```python
from build123d import *

# Parameters (mm, degrees)
SKETCH1_W           = 22
SKETCH1_H           = 13
BOSS_EXTRUDE1_DEPTH = 6
BOSS_EXTRUDE2_DEPTH = 2
BOSS_EXTRUDE3_DEPTH = 8
SKETCH4_R           = 1.525
SKETCH4_R_2         = 1.524
CUT_EXTRUDE1_DEPTH  = 36.566838488
SKETCH5_W           = 9
SKETCH5_H           = 4.088652256
CUT_EXTRUDE2_DEPTH  = 38.735924528
FILLET1_R           = 2
SKETCH6_W           = 12
SKETCH6_H           = 13.009000019
SKETCH6_W_2         = 15.838286437
CUT_EXTRUDE3_DEPTH  = 4
SKETCH7_W           = 2.5
SKETCH7_H           = 8
BOSS_EXTRUDE5_DEPTH = 3
FILLET3_R           = 2.5
FILLET4_R           = 2.5


with BuildPart() as part:
    # Sketch1 → Boss-Extrude1 (new body)
    with BuildSketch(Plane(origin=(0, 0, 0), x_dir=(1, 0, 0), z_dir=(0, 1, 0))):
        with BuildLine():
            Line((-1, -3), (23, -3))
            Line((23, -3), (25, -3))
            Line((25, -3), (25, -1))
            Line((25, -1), (25, 14))
            Line((25, 14), (25, 16))
            Line((25, 16), (23, 16))
            Line((23, 16), (-1, 16))
            ThreePointArc((-1, 16), (-2.414213562, 15.414213562), (-3, 14))
            Line((-3, 14), (-3, -1))
            ThreePointArc((-3, -1), (-2.414213562, -2.414213562), (-1, -3))
        make_face()
        with Locations((11, 6.5)):
            Rectangle(SKETCH1_W, SKETCH1_H, mode=Mode.SUBTRACT)
    extrude(amount=BOSS_EXTRUDE1_DEPTH)

    # Sketch2 → Boss-Extrude2 (add)
    with BuildSketch(Plane(origin=(0, 6, 0), x_dir=(1, 0, 0), z_dir=(0, 1, 0))):
        with BuildLine():
            Line((25, 14), (25, -1))
            Line((25, -1), (25, -3))
            Line((25, -3), (23, -3))
            Line((23, -3), (-1, -3))
            ThreePointArc((-1, -3), (-2.414213562, -2.414213562), (-3, -1))
            Line((-3, -1), (-3, 14))
            ThreePointArc((-3, 14), (-2.414213562, 15.414213562), (-1, 16))
            Line((-1, 16), (23, 16))
            Line((23, 16), (25, 16))
            Line((25, 16), (25, 14))
        make_face()
    extrude(amount=BOSS_EXTRUDE2_DEPTH)

    # Sketch3 → Boss-Extrude3 (add)
    with BuildSketch(Plane.XZ):
        with BuildLine():
            Line((5, 3), (17, 3))
            Line((17, 3), (17, 5.5))
            ThreePointArc((17, 5.5), (15.389087297, 9.389087297), (11.5, 11))
            Line((11.5, 11), (10.5, 11))
            ThreePointArc((10.5, 11), (6.610912703, 9.389087297), (5, 5.5))
            Line((5, 5.5), (5, 3))
        make_face()
        with BuildLine():
            Line((17, -16), (5, -16))
            Line((5, -16), (5, -18.5))
            ThreePointArc((5, -18.5), (6.610912703, -22.389087297), (10.5, -24))
            Line((10.5, -24), (11.5, -24))
            ThreePointArc((11.5, -24), (15.389087297, -22.389087297), (17, -18.5))
            Line((17, -18.5), (17, -16))
        make_face()
    extrude(amount=-BOSS_EXTRUDE3_DEPTH)

    # Sketch4 → Cut-Extrude1 (cut, through all)
    with BuildSketch(Plane(origin=(0, 0, 0), x_dir=(-1, 0, 0), z_dir=(0, -1, 0))):
        with Locations(Location((-11, 20, 0), (0, 0, 90))):
            Circle(SKETCH4_R)
        with Locations(Location((-11, -7, 0), (0, 0, 90))):
            Circle(SKETCH4_R_2)
    extrude(amount=-CUT_EXTRUDE1_DEPTH, mode=Mode.SUBTRACT)

    # Sketch5 → Cut-Extrude2 (cut, through all)
    with BuildSketch(Plane(origin=(25, 0, 0), x_dir=(0, 0, -1), z_dir=(1, 0, 0))):
        with Locations((6.5, 2.044326128)):
            Rectangle(SKETCH5_W, SKETCH5_H)
    extrude(amount=-CUT_EXTRUDE2_DEPTH, mode=Mode.SUBTRACT)

    # Fillet1
    fillet1_edges = [part.edges().sort_by_distance(p)[0] for p in [
        (-1.5, 4.088652256, -11),
        (-1.5, 4.088652256, -2),
        (23.5, 4.088652256, -11),
        (23.5, 4.088652256, -2),
    ]]
    fillet(fillet1_edges, radius=FILLET1_R)

    # Sketch6 → Cut-Extrude3 (cut)
    with BuildSketch(Plane(origin=(0, 8, 0), x_dir=(1, 0, 0), z_dir=(0, 1, 0))):
        with Locations((11, 22.504500009)):
            Rectangle(SKETCH6_W, SKETCH6_H)
        with Locations((11.149066226, -9.50450001)):
            Rectangle(SKETCH6_W_2, SKETCH6_H)
    extrude(amount=-CUT_EXTRUDE3_DEPTH, mode=Mode.SUBTRACT)

    # Sketch7 → Boss-Extrude5 (add)
    with BuildSketch(Plane(origin=(25, 0, 0), x_dir=(0, 0, -1), z_dir=(1, 0, 0))):
        with Locations((17.25, 4)):
            Rectangle(SKETCH7_W, SKETCH7_H)
        with Locations((-4.25, 4)):
            Rectangle(SKETCH7_W, SKETCH7_H)
    extrude(amount=-BOSS_EXTRUDE5_DEPTH)

    # Fillet3
    fillet3_edges = [part.edges().sort_by_distance(p)[0] for p in [
        (22, 4, -16),
    ]]
    fillet(fillet3_edges, radius=FILLET3_R - 0.0001)  # a hair under: the kernel refuses the full size

    # Fillet4
    fillet4_edges = [part.edges().sort_by_distance(p)[0] for p in [
        (22, 4, 3),
    ]]
    fillet(fillet4_edges, radius=FILLET4_R - 0.0001)  # a hair under: the kernel refuses the full size


solid = part.part
```
Could you check a few things on this model? Use its own coordinates, in mm. A direction names the side the tool comes from. Give positions to 0.01 mm unless a question says otherwise; leave off trailing zeros. Order: outer loops, then holes, each group sorted by start corner. A loop starts at its lowest first (then second) coordinate and runs counter-clockwise, first axis right, second up.
Q1. I'm going to push flat-ended pins straight in: P1, Ø0.6, axis at x = 23.5, y = 0.5, coming from the -Z side; P2, Ø2.5, axis at x = 11, z = 7, coming from the +Y side; P3, Ø1.5, axis at x = 1, y = 3, coming from the +Z side; P4, Ø1, axis at y = 6, z = 4, coming from the -X side. Where does each tip first touch, or does it pass through?
Q2. Suppose I cut it at C-C, the plane z = -20. Write out the boundary of the cut face in (x, y) (1 decimal).
Q3. Suppose I cut it at A-A, the plane x = 11. Write out the boundary of the cut face in (y, z) (3 decimals).
Q4. If I drill on line 1 along Z through (x, y) = (11.5, 4.25); line 2 along Z through (x, y) = (10, 0.75); line 3 along Z through (x, y) = (-0.5, 5.75), over which ranges is the centre line in solid material (lowest first)?
Q5. Suppose I cut it at D-D, the plane y = 1.25. Count the separate pieces of the cut face and the enclosed holes in it, and give its area (3 significant figures).
Q6. For faces 5 (the flat face through (9.58, 4, 6.06)), 6 (the flat face through (24, 4.089, -6)), 7 (the flat face through (17, 2, -17)), 8 (the flat face through (24, 4, -18.5)), which set-ups out of +Z, -Z, +X, -X, +Y, -Y let a thin tool reach every point of the face, with its end or its side?
Q7. We'd pull the mould along X, two halves only. Please class faces 1 (the flat face through (11, 6, -7)), 2 (the cylindrical face through (11.458, 1.972, 5.546)), 3 (the flat face through (5, 2, 4)), 4 (the flat face through (-1, 1, -11)): +X half, -X half, draft (parallel to the pull), parting line (faces both ways), or undercut.
Solution:
1. P1: stops at z = -18.5
1. P2: passes through
1. P3: stops at z = 3
1. P4: stops at x = 21
2. outline: (5.2, 0) - (9.5, 0) - (9.5, 4) - (5.2, 4) - close; (12.5, 0) - (16.8, 0) - (16.8, 4) - (12.5, 4) - close
3. outline: (0, -24) - (4, -24) - (4, -21.525) - (0, -21.525) - close; (0, -18.475) - (4, -18.475) - (4, -16) - (8, -16) - (8, 3) - (4, 3) - (4, 5.476) - (0, 5.476) - (0, 0) - (6, 0) - (6, -13) - (0, -13) - close; (0, 8.524) - (4, 8.524) - (4, 11) - (0, 11) - close
4. line 1: z = -16 to -13, 0 to 3
4. line 2: z = -23.98 to -21.15, -18.85 to -13, 0 to 5.85, 8.15 to 10.98
4. line 3: z = -16 to 3
5. separate pieces: 2
5. enclosed holes: 2
5. area: 359 mm2
6. face 5: +Z, -X, +Y
6. face 6: +X, -X, -Y
6. face 7: -Z, +Y, -Y
6. face 8: -Z, +X, +Y, -Y
7. face 1: undercut
7. face 2: undercut
7. face 3: -X half
7. face 4: draft
